Check sheet for the modelled part. Datum: model origin and axes. Units: mm. Coordinates: 2 decimals unless noted, no trailing zeros. Order: outer loops, then holes, each group sorted by start corner. A loop starts at its lowest first (then second) coordinate and runs counter-clockwise, first axis right, second up. Notation, with made-up numbers: (14, 73.5) -> (27, 73.5) arc R24 cw to (27, 105.5) -> close; hole circle Ø7 at (-27.75, 40.25). An arc over 180 degrees is marked (long way). Put each result on its own line as item: value. Start each with the question number.
```python
from build123d import *

# Parameters (mm, degrees)
SKETCH1_W           = 3.175
SKETCH1_H           = 24.635
BOSS_EXTRUDE1_DEPTH = 3.175


with BuildPart() as part:
    # Sketch1 → Boss-Extrude1 (new body)
    with BuildSketch(Plane.XY):
        Polygon((0, 0), (313, 0), (313, 24.635), (309.825, 24.635), (309.825, 49.27), (313, 49.27), (313, 73.905), (309.825, 73.905), (309.825, 98.54), (313, 98.54), (313, 123.175), (278.222222222, 123.175), (278.222222222, 120), (243.444444444, 120), (243.444444444, 123.175), (208.666666667, 123.175), (208.666666667, 120), (173.888888889, 120), (173.888888889, 123.175), (139.111111111, 123.175), (139.111111111, 120), (104.333333333, 120), (104.333333333, 123.175), (69.555555556, 123.175), (69.555555556, 120), (34.777777778, 120), (34.777777778, 123.175), (0, 123.175), (0, 98.54), (3.175, 98.54), (3.175, 73.905), (0, 73.905), (0, 49.27), (3.175, 49.27), (3.175, 24.635), (0, 24.635), align=None)
        with Locations((104.333333333, 86.2225)):
            Rectangle(SKETCH1_W, SKETCH1_H, mode=Mode.SUBTRACT)
        with Locations((104.333333333, 36.9525)):
            Rectangle(SKETCH1_W, SKETCH1_H, mode=Mode.SUBTRACT)
        with Locations((208.666666667, 86.2225)):
            Rectangle(SKETCH1_W, SKETCH1_H, mode=Mode.SUBTRACT)
        with Locations((208.666666667, 36.9525)):
            Rectangle(SKETCH1_W, SKETCH1_H, mode=Mode.SUBTRACT)
    extrude(amount=BOSS_EXTRUDE1_DEPTH)


solid = part.part
```
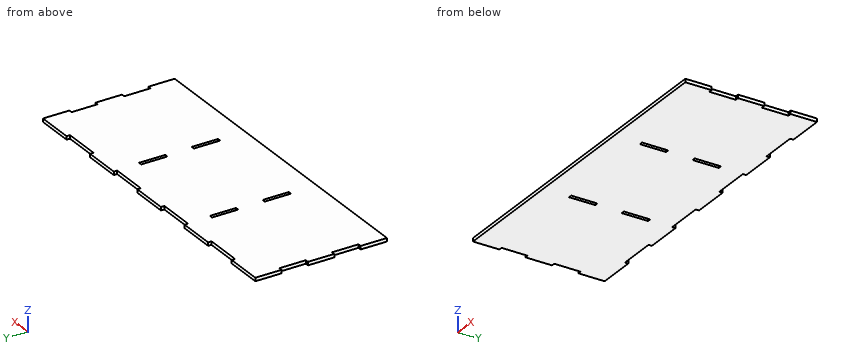
1) Sectioned sample at C-C (z = 0.95). State how many separate pieces and enclosed holes the cut face has, plus the area to 3 significant figures.
2) Gauge pin test, flat ends, axial feed: pin 1 (1.6 mm diameter, centred on y = 33, z = 2, fed in from +X) (3 decimals); pin 2 (1.6 mm diameter, centred on y = 40.5, z = 2.5, fed in from -X) (3 decimals); pin 3 (1 mm diameter, centred on x = 58.5, z = 1, fed in from +Y). Record the tip position at first contact, or that the pin passes through.
3) Sectioned sample at B-B (x = 58). Record the boundary of the cut face in (y, z) (3 decimals), plus the area to 3 significant figures.
4) Scan lines: line 1 along X through (y, z) = (39.5, 1.3) (3 decimals); line 2 along Y through (x, z) = (103.5, 0.3) (3 decimals); line 3 along Y through (x, z) = (274, 2.05). Record each from-to range of solid material in increasing order. Write a range as [from, to].
5) Sectioned sample at A-A (y = 44). Record the boundary of the cut face in (x, z) (3 decimals), plus the area to 3 significant figures.
Entries:
1. separate pieces: 1
1. enclosed holes: 4
1. area: 37,500 mm2
2. pin 1: stops at x = 309.825
2. pin 2: stops at x = 3.175
2. pin 3: stops at y = 120
3. outline: (0, 0) -> (120, 0) -> (120, 3.175) -> (0, 3.175) -> close
3. area: 381 mm2
4. line 1: x = [3.175, 102.746], [105.921, 207.079], [210.254, 309.825]
4. line 2: y = [0, 24.635], [49.27, 73.905], [98.54, 123.175]
4. line 3: y = [0, 120]
5. outline: (3.175, 0) -> (102.746, 0) -> (102.746, 3.175) -> (3.175, 3.175) -> close; (105.921, 0) -> (207.079, 0) -> (207.079, 3.175) -> (105.921, 3.175) -> close; (210.254, 0) -> (309.825, 0) -> (309.825, 3.175) -> (210.254, 3.175) -> close
5. area: 953 mm2
